Geometry: final body of the model. Coordinates: model frame, mm. Round coordinates to 2 decimals unless told otherwise and drop trailing zeros. Order: outer loops, then holes, each group sorted by start corner. A loop starts at its lowest first (then second) coordinate and runs counter-clockwise, first axis right, second up. Notation, with made-up numbers: M 20.25,40.5 L 61.25,40.5 A21 ccw 61.25,56.5 Z; hole C 54,18.25 d7. An arc over 180 degrees is marked long. Put each result on its own line as item: value. Start each with the question number.
1) First-contact query: P1, Ø4, axis at x = -95, z = 145, coming from the -Y side; P2, Ø5.5, axis at x = 95, z = -5, coming from the -Y side. Flat tips, straight axial feed; report the tip coordinate or a pass-through.
2) Section B-B, the plane y = 0.6. Count the separate pieces of the cut face and the enclosed holes in it, then the cut area to 3 significant figures.
3) Section A-A, the plane z = 15. Return loops of the section in (x, y) (3 decimals).
4) Material intervals for probe 1 along Z at (x, y) = (-85, 2.8); probe 2 along X at (y, z) = (1.4, 38); probe 3 along X at (y, z) = (1.35, 100), sorted ascending. Write a range as [from, to].
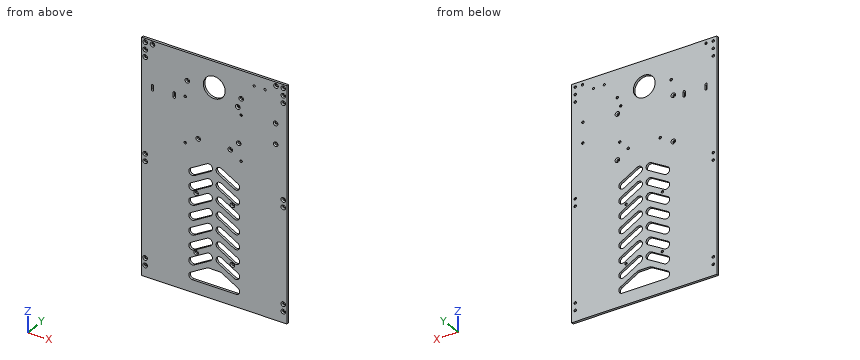
from build123d import *

# Parameters (mm, degrees)
SKETCH1_W                                       = 200
SKETCH1_H                                       = 320
BOSS_EXTRUDE1_DEPTH                             = 3.175
CSK_FOR_M3_FLAT_HEAD_MACHINE_SCREW1_D           = 3.4
CSK_FOR_M3_FLAT_HEAD_MACHINE_SCREW1_CSINK_D     = 6.3
CSK_FOR_M3_FLAT_HEAD_MACHINE_SCREW1_CSINK_ANGLE = 90
CSK_FOR_M3_FLAT_HEAD_MACHINE_SCREW2_D           = 3.4
CSK_FOR_M3_FLAT_HEAD_MACHINE_SCREW2_CSINK_D     = 6.3
CSK_FOR_M3_FLAT_HEAD_MACHINE_SCREW2_CSINK_ANGLE = 90
CSK_FOR_M3_FLAT_HEAD_MACHINE_SCREW3_D           = 3.4
CSK_FOR_M3_FLAT_HEAD_MACHINE_SCREW3_CSINK_D     = 6.3
CSK_FOR_M3_FLAT_HEAD_MACHINE_SCREW3_CSINK_ANGLE = 90
CUT_EXTRUDE1_DEPTH                              = 4.175
LPATTERN1_COUNT                                 = 8
LPATTERN1_PITCH                                 = 20
SKETCH9_R                                       = 15
SKETCH9_R_2                                     = 1.5
CUT_EXTRUDE2_DEPTH                              = 4.175
CSK_FOR_M3_FLAT_HEAD_MACHINE_SCREW4_D           = 3.4
CSK_FOR_M3_FLAT_HEAD_MACHINE_SCREW4_CSINK_D     = 6.3
CSK_FOR_M3_FLAT_HEAD_MACHINE_SCREW4_CSINK_ANGLE = 90
CSK_FOR_M3_FLAT_HEAD_MACHINE_SCREW5_D           = 3.4
CSK_FOR_M3_FLAT_HEAD_MACHINE_SCREW5_CSINK_D     = 6.3
CSK_FOR_M3_FLAT_HEAD_MACHINE_SCREW5_CSINK_ANGLE = 90


with BuildPart() as part:
    # Sketch1 → Boss-Extrude1 (new body)
    with BuildSketch(Plane(origin=(0, 0, 0), x_dir=(1, 0, 0), z_dir=(0, 1, 0))):
        Rectangle(SKETCH1_W, SKETCH1_H)
    extrude(amount=BOSS_EXTRUDE1_DEPTH)

    # CSK for M3 Flat Head Machine Screw1 (through all)
    with Locations(Plane.XZ):
        with Locations((-95, 155), (-85, 155), (-95, 145), (-95, 135), (-95, -145), (-95, -135), (-95, 5), (-95, -5)):
            csk_for_m3_flat_head_machine_screw1 = CounterSinkHole(CSK_FOR_M3_FLAT_HEAD_MACHINE_SCREW1_D / 2, CSK_FOR_M3_FLAT_HEAD_MACHINE_SCREW1_CSINK_D / 2, counter_sink_angle=CSK_FOR_M3_FLAT_HEAD_MACHINE_SCREW1_CSINK_ANGLE)

    # Mirror1: CSK for M3 Flat Head Machine Screw1 across plane
    add(csk_for_m3_flat_head_machine_screw1.mirror(Plane(origin=(0, 0, 0), x_dir=(0, 0, 1), z_dir=(1, 0, 0))), mode=Mode.SUBTRACT)

    # CSK for M3 Flat Head Machine Screw2 (through all)
    with Locations(Plane.XZ):
        with Locations((-25, -105), (25, -105), (25, -25), (-25, -25)):
            CounterSinkHole(CSK_FOR_M3_FLAT_HEAD_MACHINE_SCREW2_D / 2, CSK_FOR_M3_FLAT_HEAD_MACHINE_SCREW2_CSINK_D / 2, counter_sink_angle=CSK_FOR_M3_FLAT_HEAD_MACHINE_SCREW2_CSINK_ANGLE)

    # CSK for M3 Flat Head Machine Screw3 (through all)
    with Locations(Plane(origin=(0, 3.175, 0), x_dir=(-1, 0, 0), z_dir=(0, 1, 0))):
        with Locations((40, 38), (-37, 100), (-37, 38), (40, 100)):
            CounterSinkHole(CSK_FOR_M3_FLAT_HEAD_MACHINE_SCREW3_D / 2, CSK_FOR_M3_FLAT_HEAD_MACHINE_SCREW3_CSINK_D / 2, counter_sink_angle=CSK_FOR_M3_FLAT_HEAD_MACHINE_SCREW3_CSINK_ANGLE)

    # Sketch8 → Cut-Extrude1 (cut, through all)
    with BuildSketch(Plane(origin=(0, 3.175, 0), x_dir=(1, 0, 0), z_dir=(0, 1, 0))):
        with BuildLine():
            Line((-10, -19.330127019), (-32.5, -6.339745962))
            ThreePointArc((-32.5, -6.339745962), (-34.330127019, 0.490381057), (-27.5, 2.320508076))
            Line((-27.5, 2.320508076), (-5, -10.669872981))
            ThreePointArc((-5, -10.669872981), (-3.169872981, -17.5), (-10, -19.330127019))
        make_face()
        with BuildLine():
            Line((10, -19.330127019), (32.5, -6.339745962))
            ThreePointArc((32.5, -6.339745962), (34.330127019, 0.490381057), (27.5, 2.320508076))
            Line((27.5, 2.320508076), (5, -10.669872981))
            ThreePointArc((5, -10.669872981), (3.169872981, -17.5), (10, -19.330127019))
        make_face()
    cut_extrude1 = extrude(amount=-CUT_EXTRUDE1_DEPTH, mode=Mode.SUBTRACT)

    # LPattern1: Cut-Extrude1 ×8
    with Locations(*[(0, 0, -i * LPATTERN1_PITCH) for i in range(1, LPATTERN1_COUNT)]):
        add(cut_extrude1, mode=Mode.SUBTRACT)

    # Sketch9 → Cut-Extrude2 (cut, through all)
    with BuildSketch(Plane(origin=(0, 3.175, 0), x_dir=(1, 0, 0), z_dir=(0, 1, 0))):
        with Locations((0, -125)):
            Circle(SKETCH9_R)
        with Locations((55, -145)):
            Circle(SKETCH9_R_2)
        with Locations((70, -145)):
            Circle(SKETCH9_R_2)
        with BuildLine():
            Line((-7.5, 120), (7.5, 120))
            ThreePointArc((7.5, 120), (8.794095226, 120.170370869), (10, 120.669872981))
            Line((10, 120.669872981), (32.5, 133.660254038))
            ThreePointArc((32.5, 133.660254038), (34.829629131, 139.284476282), (30, 142.990381057))
            Line((30, 142.990381057), (-30, 142.990381057))
            ThreePointArc((-30, 142.990381057), (-34.829629131, 139.284476282), (-32.5, 133.660254038))
            Line((-32.5, 133.660254038), (-10, 120.669872981))
            ThreePointArc((-10, 120.669872981), (-8.794095226, 120.170370869), (-7.5, 120))
        make_face()
        with BuildLine():
            Line((-83.5, -94), (-83.5, -100))
            ThreePointArc((-83.5, -100), (-85, -101.5), (-86.5, -100))
            Line((-86.5, -100), (-86.5, -94))
            ThreePointArc((-86.5, -94), (-85, -92.5), (-83.5, -94))
        make_face()
        with BuildLine():
            Line((-56.5, -94), (-56.5, -100))
            ThreePointArc((-56.5, -100), (-55, -101.5), (-53.5, -100))
            Line((-53.5, -100), (-53.5, -94))
            ThreePointArc((-53.5, -94), (-55, -92.5), (-56.5, -94))
        make_face()
    extrude(amount=-CUT_EXTRUDE2_DEPTH, mode=Mode.SUBTRACT)

    # CSK for M3 Flat Head Machine Screw4 (through all)
    with Locations(Plane.XZ):
        with Locations((84.46, 104.38), (32.39, 109.46), (33.66, 61.2), (84.46, 76.44)):
            CounterSinkHole(CSK_FOR_M3_FLAT_HEAD_MACHINE_SCREW4_D / 2, CSK_FOR_M3_FLAT_HEAD_MACHINE_SCREW4_CSINK_D / 2, counter_sink_angle=CSK_FOR_M3_FLAT_HEAD_MACHINE_SCREW4_CSINK_ANGLE)

    # CSK for M3 Flat Head Machine Screw5 (through all)
    with Locations(Plane.XZ):
        with Locations((-37, 122), (37, 122), (22, 48.822134494), (-22, 48.822134494)):
            CounterSinkHole(CSK_FOR_M3_FLAT_HEAD_MACHINE_SCREW5_D / 2, CSK_FOR_M3_FLAT_HEAD_MACHINE_SCREW5_CSINK_D / 2, counter_sink_angle=CSK_FOR_M3_FLAT_HEAD_MACHINE_SCREW5_CSINK_ANGLE)


solid = part.part
Result sheet:
1. P1: stops at y = 1.15
1. P2: stops at y = 0.4
2. separate pieces: 1
2. enclosed holes: 52
2. area: 56,700 mm2
3. outline: M -100,0 L -17.5,0 L -17.5,3.175 L -100,3.175 Z; M -2.5,0 L 2.5,0 L 2.5,3.175 L -2.5,3.175 Z; M 17.5,0 L 100,0 L 100,3.175 L 17.5,3.175 Z
4. probe 1: z = [-160, 92.5], [101.5, 153.3], [156.7, 160]
4. probe 2: x = [-100, -41.7], [-38.3, 35.3], [38.7, 100]
4. probe 3: x = [-100, -86.5], [-83.5, -56.5], [-53.5, -41.7], [-38.3, 35.3], [38.7, 100]
